```python
from build123d import *

# Parameters (mm, degrees)
F0_R      = 26.0530381456
F0_R_2    = 24.5437010233
F1_DEPTH  = 50.8
F2_W      = 37.793032825
F2_H      = 48.0312788859
F3_DEPTH  = 50.8
F7_START  = 48.768
F6_R      = 26.0407706564
F7_DEPTH  = 1.778
F9_START  = -49.276
F8_R      = 26.1069464333
F9_DEPTH  = 1.27
F10_R     = 2.063301756
F11_DEPTH = 50.8
F12_R     = 1.8097447332
F13_DEPTH = 50.8


# Not quite as in the source:
# - the program builds the solid bodies; features that only make, move or delete a surface that nothing else refers to are left out


with BuildPart() as f1:
    # F0 (on Front) → F1 (new body, symmetric)
    with BuildSketch(Plane.XZ):
        Circle(F0_R)
        Circle(F0_R_2, mode=Mode.SUBTRACT)
    extrude(amount=F1_DEPTH, both=True)

    # F2 (on Front) → F3 (cut, symmetric)
    with BuildSketch(Plane.XZ):
        with Locations((18.8965164125, 11.3758291118)):
            Rectangle(F2_W, F2_H)
    extrude(amount=F3_DEPTH, both=True, mode=Mode.SUBTRACT)

    # F6 (on Front) → F7 (join)
    with BuildSketch(Plane.XZ.offset(F7_START)):
        Circle(F6_R)
    extrude(amount=F7_DEPTH)

    # F8 (on Front) → F9 (join)
    with BuildSketch(Plane.XZ.offset(F9_START)):
        Circle(F8_R)
    extrude(amount=-F9_DEPTH)

    # F10 (on Front) → F11 (join, symmetric)
    with BuildSketch(Plane.XZ):
        with Locations((0, 19.7181049734)):
            Circle(F10_R)
    extrude(amount=F11_DEPTH, both=True)

    # F12 (on Front) → F13 (cut, symmetric)
    with BuildSketch(Plane.XZ):
        Circle(F12_R)
    extrude(amount=F13_DEPTH, both=True, mode=Mode.SUBTRACT)


solid = f1.part
```
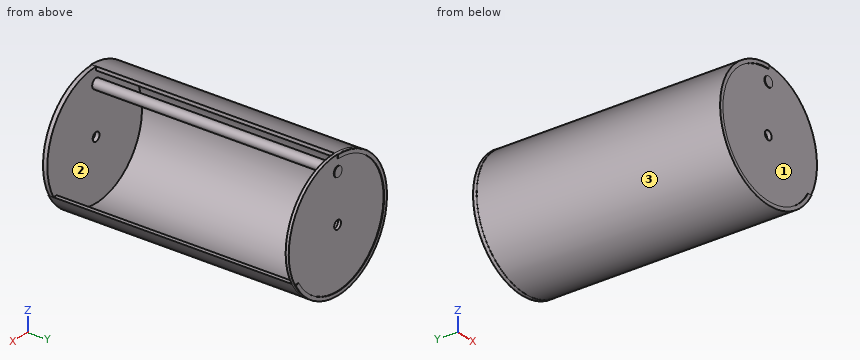
CAD build for the part. Positions are in the model's coordinates, mm. Face numbers are marked on the shaded views. Give positions to 0.01 mm unless a question says otherwise; leave off trailing zeros. Order: outer loops, then holes, each group sorted by start corner. A loop starts at its lowest first (then second) coordinate and runs counter-clockwise, first axis right, second up. Notation, with made-up numbers: M 62.25,-22 L 89.25,-22 A13 cw 89.25,-14 Z; hole C 37.25,-10.75 d10. An arc over 180 degrees is marked long. Put each result on its own line as item: value. Start each with the question number.
(1) Saw through at C-C, the plane z = -18. Write the cut outline in (x, y), then the cut area to 3 significant figures.
(2) Saw through at B-B, the plane x = -22.5. Write the cut outline in (y, z).
(3) Flat gauge pins, fed straight in: pin 1 Ø0.5 at (y, z) = (11, 25.5) entering from +X; pin 2 Ø10 at (x, y) = (0.5, 35.5) entering from +Z; pin 3 Ø3.5 at (x, z) = (0, 0) entering from +Y; pin 4 Ø1 at (y, z) = (40.5, 11.5) entering from +X. Where does each tip first touch, or does it go through?
(4) Saw through at D-D, the plane y = -20.5. Write the cut outline in (x, z).
(5) Mould opens along Z. For the marked faces 1, 2 and 3 say: +Z half, -Z half, draft (parallel to the pull), parting line (faces both ways), or undercut.
(6) Saw through at A-A, the plane z = 0. Write the cut outline in (x, y), then the cut area to 3 significant figures.
(7) Drill centre lines: line 1 along Y through (x, z) = (-5, 8); line 2 along Z through (x, y) = (-18, 1); line 3 along X through (y, z) = (-6, 0). Where is each one in solid material? Low to high.
Check result:
1. outline: M -18.91,49.28 L -18.84,49.28 L -18.84,-50.8 L -16.69,-50.8 L -16.69,-50.55 L 16.69,-50.55 L 16.69,-50.8 L 18.84,-50.8 L 18.84,49.28 L 18.91,49.28 L 18.91,50.55 L 18.84,50.55 L 18.84,50.8 L 16.69,50.8 L 16.69,50.55 L -16.69,50.55 L -16.69,50.8 L -18.84,50.8 L -18.84,50.55 L -18.91,50.55 Z; hole M -16.69,-48.77 L 16.69,-48.77 L 16.69,49.28 L -16.69,49.28 Z
1. area: 539 mm2
2. outline: M -50.8,-13.13 L 49.28,-13.13 L 49.28,-13.24 L 50.55,-13.24 L 50.55,-13.13 L 50.8,-13.13 L 50.8,-9.81 L 50.55,-9.81 L 50.55,9.81 L 50.8,9.81 L 50.8,13.13 L 50.55,13.13 L 50.55,13.24 L 49.28,13.24 L 49.28,13.13 L -50.8,13.13 L -50.8,9.81 L -50.55,9.81 L -50.55,-9.81 L -50.8,-9.81 Z; hole M -48.77,-9.81 L 49.28,-9.81 L 49.28,9.81 L -48.77,9.81 Z
3. pin 1: stops at x = 0
3. pin 2: stops at z = 26.05
3. pin 3: passes through
3. pin 4: stops at x = -21.41
4. outline: C 0,19.72 d4.13; M 0,24.54 L 0,26.05 A26.05 ccw long 22.78,-12.64 L 21.04,-12.64 A24.54 cw long Z
5. face 1: undercut
5. face 2: undercut
5. face 3: parting line
6. outline: M -26.11,49.28 L -26.05,49.28 L -26.05,-50.8 L -24.54,-50.8 L -24.54,-50.55 L -1.81,-50.55 L -1.81,-48.77 L -24.54,-48.77 L -24.54,49.28 L -1.81,49.28 L -1.81,50.55 L -24.54,50.55 L -24.54,50.8 L -26.05,50.8 L -26.05,50.55 L -26.11,50.55 Z; M 1.81,-50.55 L 26.04,-50.55 L 26.04,-48.77 L 1.81,-48.77 Z; M 1.81,49.28 L 26.11,49.28 L 26.11,50.55 L 1.81,50.55 Z
6. area: 297 mm2
7. line 1: y = -50.55 to -48.77, 49.28 to 50.55
7. line 2: z = -18.84 to -16.69, 16.69 to 18.84
7. line 3: x = -26.05 to -24.54
